CAD build for the part. Positions are in the model's coordinates, mm. Face numbers are marked on the shaded views. A direction names the side the tool comes from. Give positions to 0.01 mm unless a question says otherwise; leave off trailing zeros. Loops run counter-clockwise (first coordinate to the right, second up) from the corner with the lowest first, then second, coordinate; pieces in that order, holes last. Notation, with made-up numbers: (29, -18) - (84, -18) arc R22 cw to (84, 10) - close; hole circle Ø9 at (8, -15.5). An arc over 180 degrees is marked (long way). Return JSON: item names as keys, results as strings.
Autodesk Inventor part; units mm, degrees
ref_plane "YZ Plane" through (0, 0, 0) normal (1, 0, 0) x (0, 1, 0)
ref_plane "XZ Plane" through (0, 0, 0) normal (0, 1, 0) x (-1, 0, 0)
ref_plane "XY Plane" through (0, 0, 0) normal (0, 0, 1) x (1, 0, 0)
sketch "Boceto1" plane through (0, 0, 0) normal (0, 1, 0) x (-1, 0, 0)
  circle A0 centre (0, 0) radius 1.5
  line L0 (4, 4) -> (-4, 4)
  line L1 (-4, 4) -> (-4, -4)
  line L2 (-4, -4) -> (4, -4)
  line L3 (4, -4) -> (4, 4)
  dimension "d0" = 3
extrude "Extrusión1" add sketch "Boceto1" along normal blind 2
sketch "Boceto2" plane through (-4, 0, -4) normal (-1, 0, 0) x (0, 0, 1)
  circle A0 centre (4, 6) radius 1.5
  line L0 (8, 2) -> (8, 10)
  line L1 (8, 10) -> (0, 10)
  line L2 (0, 10) -> (0, 2)
  line L3 (8, 0) -> (0, 0)
  line L4 (0, 0) -> (8, 0)
  line L5 (8, 0) -> (8, 2)
  line L6 (0, 2) -> (0, 0)
  line L7 (0, 0) -> (8, 0)
  line L8 (8, 0) -> (8, 10)
  line L9 (8, 10) -> (0, 10)
  line L10 (0, 10) -> (0, 0)
  point P0 (4, 0)
extrude "Extrusión2" add sketch "Boceto2" along normal blind 2
sketch "Boceto3" plane through (4, 0, 4) normal (0, 0, 1) x (1, 0, 0)
  line L0 (-8, 2) -> (-8, 10)
  line L1 (-8, 10) -> (-8, 8)
  line L2 (0, 2) -> (-2, 2)
  line L3 (-2, 2) -> (-8, 8)
  line L4 (-2, 2) -> (-8, 2)
  line L5 (-8, 8) -> (-8, 2)
  point P0 (-5.5, 2)
  point P1 (-8, 4.5)
  dimension "d26" = 2
  dimension "d27" = 2
extrude "Extrusión8" add sketch "Boceto3" against normal blind 2
sketch "Boceto9" plane through (4, 0, -4) normal (0, 0, -1) x (-1, 0, 0)
  line L0 (0, 2) -> (8, 2)
  line L1 (8, 8) -> (2, 2)
  line L2 (2, 2) -> (8, 8)
  line L3 (8, 8) -> (8, 2)
  line L4 (8, 2) -> (2, 2)
  point P0 (4, 0)
extrude "Extrusión9" add sketch "Boceto9" against normal blind 2
properties part number "Base auxiliar - esquadra"
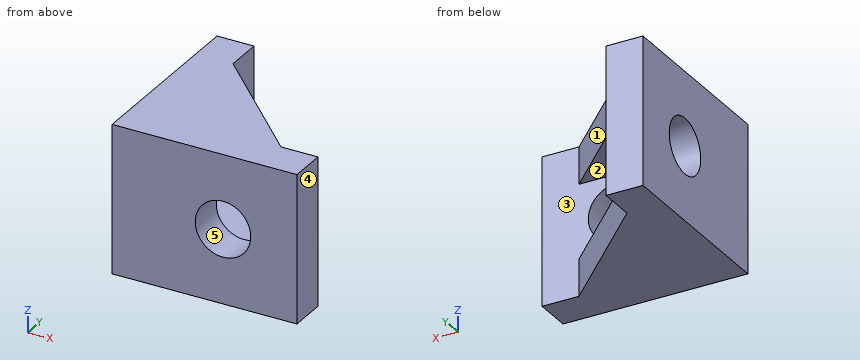
1. Cut at A-A, the plane z = 0. Write the cut outline in (x, y).
Values follow:
{"outline": "(-6, 0) - (-1.5, 0) - (-1.5, 2) - (-4, 2) - (-4, 4.5) - (-6, 4.5) - close; (-6, 7.5) - (-4, 7.5) - (-4, 10) - (-6, 10) - close; (1.5, 0) - (4, 0) - (4, 2) - (1.5, 2) - close"}
2. Drop flat-ended pins along their axis: P1, Ø1.8, axis at x = 0, z = 0, coming from the +Y side; P2, Ø4, axis at y = 6.5, z = -1.5, coming from the +X side; P3, Ø2, axis at x = 1.5, z = 0, coming from the -Y side. Give the stop position or say it passes through.
Values follow:
{"P1": "passes through", "P2": "stops at x = -0.56", "P3": "stops at y = 0"}
3. Cut at D-D, the plane x = -4.5. Write the cut outline in (y, z).
Values follow:
{"outline": "(0, -4) - (10, -4) - (10, 4) - (0, 4) - close; hole circle Ø3 at (6, 0)"}
4. Which spindle directions (+Z, -Z, +X, -X, +Y, -Y) get a long thin tool onto all of the face, cutting with end or side? Do the marked faces 1 and 2. Say none if no direction does.
Values follow:
{"face 1": "+Z, -Z, +X, +Y", "face 2": "+X, +Y"}
5. Pull direction X, two halves, no side cores. Call the marked faces 3, 4 and 5: +X half, -X half, draft (parallel to the pull), parting line (faces both ways), or undercut.
Values follow:
{"face 3": "draft", "face 4": "+X half", "face 5": "undercut"}
6. Drill centre lines: probe 1 along Z at (x, y) = (0, 1.4); probe 2 along X at (y, z) = (5, -1.5); probe 3 along Z at (x, y) = (-3, 2.75). Where is each one in solid material? Low to high.
Values follow:
{"probe 1": "z = -4 to -1.5, 1.5 to 4", "probe 2": "x = -6 to -4", "probe 3": "z = -4 to -2, 2 to 4"}
7. Cut at B-B, the plane y = 6. Write the cut outline in (x, z), plus the area to 3 significant figures.
Values follow:
{"outline": "(-6, -4) - (-2, -4) - (-2, -2) - (-4, -2) - (-4, -1.5) - (-6, -1.5) - close; (-6, 1.5) - (-4, 1.5) - (-4, 2) - (-2, 2) - (-2, 4) - (-6, 4) - close", "area": "18.0 mm²"}
8. Cut at C-C, the plane x = 0. Write the cut outline in (y, z), plus the area to 3 significant figures.
Values follow:
{"outline": "(0, -4) - (4, -4) - (4, -2) - (2, -2) - (2, -1.5) - (0, -1.5) - close; (0, 1.5) - (2, 1.5) - (2, 2) - (4, 2) - (4, 4) - (0, 4) - close", "area": "18.0 mm²"}
